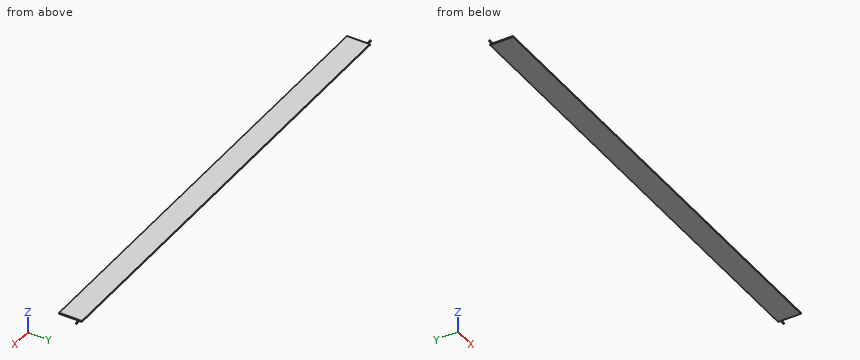
```python
from build123d import *

# Parameters (mm, degrees)
SKETCH1_W                = 1181.1
SKETCH1_H                = 57.15
BOSS_EXTRUDE1_DEPTH      = 1.27
SKETCH2_R                = 1.27
BOSS_EXTRUDE2_DEPTH      = 12.7
BOSS_EXTRUDE2_DEPTH_BACK = 1193.8


with BuildPart() as part:
    # Sketch1 → Boss-Extrude1 (new body, symmetric)
    with BuildSketch(Plane.XY):
        Rectangle(SKETCH1_W, SKETCH1_H)
    extrude(amount=BOSS_EXTRUDE1_DEPTH, both=True)

    # Sketch2 → Boss-Extrude2 (add, two sides)
    with BuildSketch(Plane.ZY.offset(590.55)) as boss_extrude2_sk:
        with Locations((0, 22.225)):
            Circle(SKETCH2_R)
    extrude(amount=BOSS_EXTRUDE2_DEPTH)
    extrude(boss_extrude2_sk.sketch, amount=-BOSS_EXTRUDE2_DEPTH_BACK)


solid = part.part
```
Could you check a few things on this model? Use its own coordinates, in mm. Coordinates: 2 decimals unless noted, no trailing zeros. Write each loop counter-clockwise with the first axis right and the second up, starting at its lowest first coordinate (ties: lowest second). Pieces come first, ordered by that corner, then holes. Notation, with made-up numbers: (84, -5.5) -> (108, -5.5) arc R19 cw to (108, 1.5) -> close; hole circle Ø1 at (50, -10.75). An arc over 180 degrees is marked (long way). Write item = value, one per line. Start each with the question number.
(1) Will these pins go through, and if not, where does the flat tip stop? pin 1 (1.3 mm diameter, centred on y = 24.5, z = -0.5, fed in from +X); pin 2 (1 mm diameter, centred on y = 13, z = -0.5, fed in from -X).
(2) I want a section at B-B (y = -9). Please give me the cut outline in (x, z).
(3) I need wall thicknesses on line 1 (X direction, y = 3, z = 1.2). Which ranges of the line are inside material? Lowest first, please. Write a range as [from, to].
(4) I want a section at A-A (z = 0). Please give me the cut outline in (x, y) (3 decimals).
Result set:
q1.pin_1 = 590.55
q1.pin_2 = -590.55
q2.outline = (-590.55, -1.27) -> (590.55, -1.27) -> (590.55, 1.27) -> (-590.55, 1.27) -> close
q3.line_1 = [-590.55, 590.55]
q4.outline = (-603.25, 20.955) -> (-590.55, 20.955) -> (-590.55, -28.575) -> (590.55, -28.575) -> (590.55, 20.955) -> (603.25, 20.955) -> (603.25, 23.495) -> (590.55, 23.495) -> (590.55, 28.575) -> (-590.55, 28.575) -> (-590.55, 23.495) -> (-603.25, 23.495) -> close
